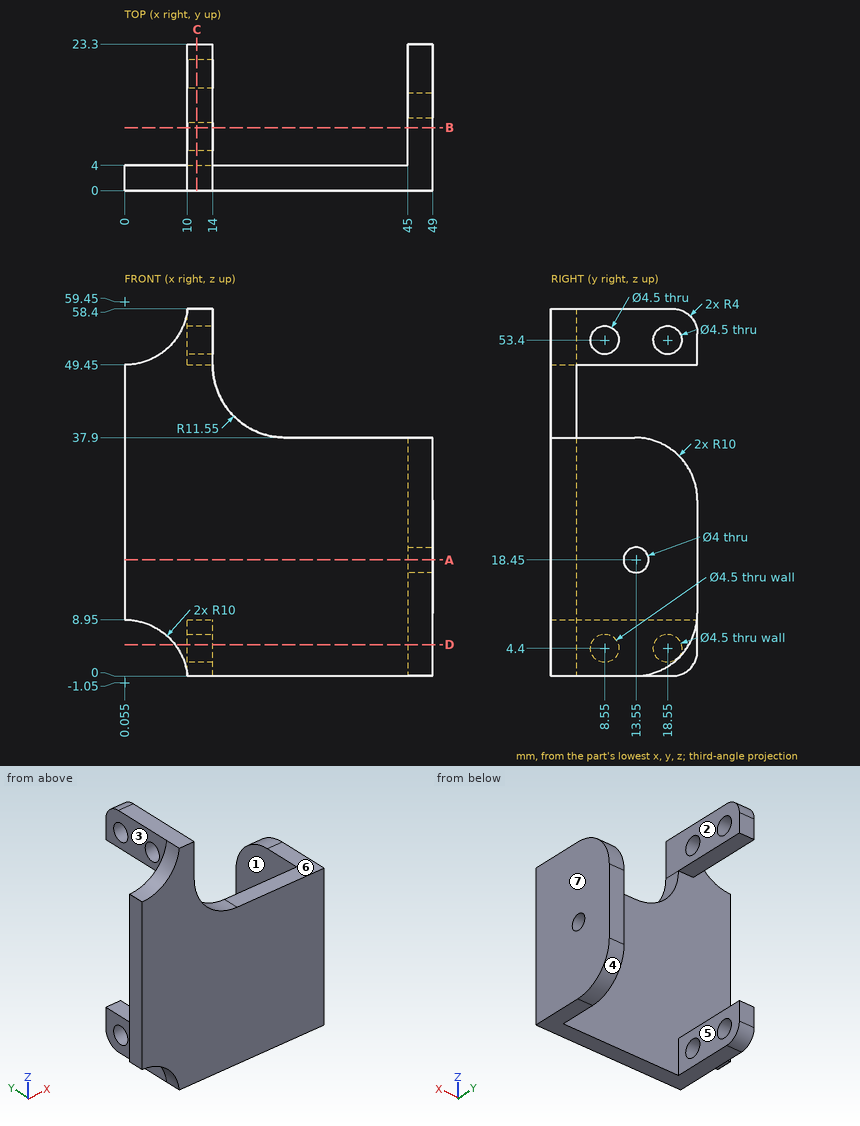
Design review of the part shown in the three views and the two pictorial views. Dimensions are in mm from the part's minimum x, y and z. A direction names the side the tool comes from. Round coordinates to 2 decimals unless told otherwise and drop trailing zeros. Write each loop counter-clockwise with the first axis right and the second up, starting at its lowest first coordinate (ties: lowest second). Pieces come first, ordered by that corner, then holes. Notation, with made-up numbers: M -26,-28.5 L -5,-28.5 A28 cw -5,-10.5 Z; hole C 11,25.5 d6. An arc over 180 degrees is marked long. Use a Markdown table: item, result. Add a question column.
Q1. The part is to be moulded in two halves that separate along X. For the marked faces 1, 2, 3 and 4, say which applies: pulls with the +X half, pulls with the -X half, needs draft (parallel to the pull), parting line crosses it, or undercut.
Q2. We need section C-C, the plane x = 11.5. State the section outline as (y, z) points.
Q3. Insertion check: pin 1 (4.5 mm diameter, centred on y = 13.55, z = 18.45, fed in from -X); pin 2 (1 mm diameter, centred on x = 6.5, y = 6, fed in from +Z) (3 decimals); pin 3 (13.5 mm diameter, centred on x = 18.5, z = 37.5, fed in from +Y); pin 4 (5 mm diameter, centred on x = 30, y = 3, fed in from +Z). Each pin has a flat end and moves straight along its axis. Give the tip position at first contact, or say it passes through.
Q4. To check wall thickness, follow line 1 (Y direction, x = 13.2, z = 4.4); line 2 (Z direction, x = 13, y = 17); line 3 (X direction, y = 18.25, z = 27). State the ranges of each line that lie inside material, in increasing order.
Q5. Machinability: for the marked faces 5, 6 and 7, which of the approach directions +Z, -Z, +X, -X, +Y, -Y give a long, thin tool a straight path to every point of the face, cutting with its end or side? Answer none if there is none.
Q6. We need section B-B, the plane y = 10. State the section outline as (x, z) points.
Q7. We need section D-D, the plane z = 5. State the section outline as (x, y) points.
Q8. We need section A-A, the plane z = 18.45. State the section outline as (x, y) points, plus the area to 3 significant figures.
Findings below:
| question | item | result |
|---|---|---|
| 1 | face 1 | undercut |
| 1 | face 2 | pulls with the +X half |
| 1 | face 3 | pulls with the -X half |
| 1 | face 4 | needs draft |
| 2 | outline | M 0,0 L 19.3,0 A4 ccw 23.3,4 L 23.3,8.95 L 4,8.95 L 4,49.45 L 23.3,49.45 L 23.3,54.4 A4 ccw 19.3,58.4 L 0,58.4 Z; hole C 8.55,4.4 d4.5; hole C 8.55,53.4 d4.5; hole C 18.55,4.4 d4.5; hole C 18.55,53.4 d4.5 |
| 3 | pin 1 | stops at x = 45 |
| 3 | pin 2 | passes through |
| 3 | pin 3 | stops at y = 4 |
| 3 | pin 4 | stops at z = 37.9 |
| 4 | line 1 | y = 0 to 6.3, 10.8 to 16.3, 20.8 to 23.3 |
| 4 | line 2 | z = 0 to 2.77, 6.03 to 8.95, 49.45 to 51.77, 55.03 to 58.4 |
| 4 | line 3 | x = 45 to 49 |
| 5 | face 5 | +Z, -Z, +Y |
| 5 | face 6 | +Z, +X, +Y, -Y |
| 5 | face 7 | +Z, -Z, +X, +Y, -Y |
| 6 | outline | M 10,0 L 14,0 L 14,2.68 L 10,2.68 Z; M 10,6.12 L 14,6.12 L 14,8.95 L 10,8.95 Z; M 10,49.45 L 14,49.45 L 14,51.68 L 10,51.68 Z; M 10,55.12 L 14,55.12 L 14,58.4 L 10,58.4 Z; M 45,0 L 49,0 L 49,37.9 L 45,37.9 Z |
| 7 | outline | M 8.02,0 L 49,0 L 49,21.96 L 45,21.96 L 45,4 L 14,4 L 14,6.38 L 10,6.38 L 10,4 L 8.02,4 Z; M 10,10.72 L 14,10.72 L 14,16.38 L 10,16.38 Z; M 10,20.72 L 14,20.72 L 14,23.3 L 10,23.3 Z |
| 8 | outline | M 0,0 L 49,0 L 49,11.55 L 45,11.55 L 45,4 L 0,4 Z; M 45,15.55 L 49,15.55 L 49,23.3 L 45,23.3 Z |
| 8 | area | 257 mm² |
